Source: CAD feature listing. Evaluate the final solid. Frame: model axes, mm. A direction names the side the tool comes from. Coordinates: 2 decimals unless noted, no trailing zeros. Order: outer loops, then holes, each group sorted by start corner. A loop starts at its lowest first (then second) coordinate and runs counter-clockwise, first axis right, second up.
Item 1: Contact query for flat-ended pins moving along their axis: P1, Ø4.5, axis at x = 1.5, y = 4, coming from the +Z side; P2, Ø3, axis at x = 10, y = 8.5, coming from the +Z side; P3, Ø1, axis at y = 14, z = -1.5, coming from the +X side; P4, Ø1.2, axis at x = 1, y = 13, coming from the -Z side. Output: stop coordinate, or through.
Item 2: Reachability of faces 1 (the flat face through (2.9, 12.5, -4.8)), 2 (the flat face through (7, 7, -36)), 3 (the flat face through (1, 14, -2)) from +Z, -Z, +X, -X, +Y, -Y: full face, straight path, thin tool, end or side. Return the list, or none.
Item 3: Section A-A on x = 21.5. Return the cut outline in (y, z), then the cut area to 3 significant figures.
Item 4: Mould query, pull axis Y, two halves, no side actions, for faces 4 (the flat face through (7.2, 7.4, -9.5)), 5 (the flat face through (6, 15, -36)), 6 (the flat face through (-2, 7, -23)). Classes: released by +Y, released by -Y, zero draft, split by the parting line, or undercut.
Item 5: Section D-D on z = -26.5. Return the cut outline in (x, y).
Item 6: Ray query, line 1 (X direction, y = 12.5, z = -26.5); line 2 (Z direction, x = 34, y = 14.5); line 3 (X direction, y = 10.75, z = -15). Return the intervals inside material, ascending.
Item 7: Section C-C on z = -46. Return the cut outline in (x, y), then the cut area to 3 significant figures.
from build123d import *

# Parameters (mm, degrees)
SKETCH2_W               = 4
SKETCH2_H               = 28.5
BOSS_EXTRUDE1_DEPTH     = 15
CUT_EXTRUDE1_DEPTH      = 86.527773267
CUT_EXTRUDE1_DEPTH_BACK = 15
SKETCH3_W               = 9.5
SKETCH3_H               = 10
FILLET1_R               = 2
FILLET2_R               = 2
FILLET3_R               = 2
FILLET4_R               = 2
FILLET5_R               = 2
FILLET6_R               = 2


with BuildPart() as part:
    # Sketch2 → Boss-Extrude1 (new body)
    with BuildSketch(Plane(origin=(0, 0, 0), x_dir=(1, 0, 0), z_dir=(0, 1, 0))):
        Polygon((0, 0), (0, 2), (2, 2), (2, 0), (4, 0), (49, 67), (4, 67), (4, 39.5), (2, 39.5), (2, 36.5), (0, 36.5), (0, 37.5), (-2, 37.5), (-2, 0), align=None)
        with Locations((2, 19.25)):
            Rectangle(SKETCH2_W, SKETCH2_H, mode=Mode.SUBTRACT)
        Polygon((7, 64), (43.371222906, 64), (7, 9.516238481), align=None, mode=Mode.SUBTRACT)
    extrude(amount=BOSS_EXTRUDE1_DEPTH)

    # Sketch3 → Cut-Extrude1 (cut, two sides: drawn at the far end of the back side and taken through both)
    with BuildSketch(Plane.ZY.offset(2).offset(-CUT_EXTRUDE1_DEPTH_BACK)):
        with Locations((-4.75, 7.5)):
            Rectangle(SKETCH3_W, SKETCH3_H)
    extrude(amount=CUT_EXTRUDE1_DEPTH + CUT_EXTRUDE1_DEPTH_BACK, mode=Mode.SUBTRACT)

    # Fillet1
    fillet1_edges = [part.edges().sort_by_distance(p)[0] for p in [
        (-2, 7.5, -37.5),
    ]]
    fillet(fillet1_edges, radius=FILLET1_R - 0.0001)  # a hair under: the kernel refuses the full size

    # Fillet2
    fillet2_edges = [part.edges().sort_by_distance(p)[0] for p in [
        (4, 7.5, -67),
    ]]
    fillet(fillet2_edges, radius=FILLET2_R)

    # Fillet3
    fillet3_edges = [part.edges().sort_by_distance(p)[0] for p in [
        (4, 1.25, 0),
    ]]
    fillet(fillet3_edges, radius=FILLET3_R)

    # Fillet4
    fillet4_edges = [part.edges().sort_by_distance(p)[0] for p in [
        (4, 13.75, 0),
    ]]
    fillet(fillet4_edges, radius=FILLET4_R)

    # Fillet5
    fillet5_edges = [part.edges().sort_by_distance(p)[0] for p in [
        (-2, 13.75, 0),
    ]]
    fillet(fillet5_edges, radius=FILLET5_R - 0.0001)  # a hair under: the kernel refuses the full size

    # Fillet6
    fillet6_edges = [part.edges().sort_by_distance(p)[0] for p in [
        (-2, 1.25, 0),
    ]]
    fillet(fillet6_edges, radius=FILLET6_R - 0.0001)  # a hair under: the kernel refuses the full size


solid = part.part
Answer list:
1. P1: stops at z = 0
1. P2: stops at z = -9.5
1. P3: stops at x = 5.34
1. P4: stops at z = -36.5
2. face 1: +Z, +X, -X
2. face 2: +Y, -Y
2. face 3: +Z, +Y, -Y
3. outline: (0, -67) - (15, -67) - (15, -64) - (0, -64) - close; (0, -31.24) - (15, -31.24) - (15, -26.06) - (0, -26.06) - close
3. area: 123 mm2
4. face 4: undercut
4. face 5: released by +Y
4. face 6: zero draft
5. outline: (-2, 0) - (0, 0) - (0, 15) - (-2, 15) - close; (4, 0) - (7, 0) - (7, 15) - (4, 15) - close; (18.34, 0) - (21.8, 0) - (21.8, 15) - (18.34, 15) - close
6. line 1: x = -2 to 0, 4 to 7, 18.34 to 21.8
6. line 2: z = -67 to -64, -49.96 to -44.67
6. line 3: x = -2 to 0, 4 to 7, 10.66 to 14.07
7. outline: (4, 0) - (7, 0) - (7, 15) - (4, 15) - close; (31.36, 0) - (34.9, 0) - (34.9, 15) - (31.36, 15) - close
7. area: 98.1 mm2
